Input: dimensioned drawing with shaded views. Units: mm. Origin: part minimum x, y, z. Give positions to 0.01 mm unless a question says otherwise; leave off trailing zeros. Loops run counter-clockwise (first coordinate to the right, second up) from the corner with the lowest first, then second, coordinate; pieces in that order, holes last.
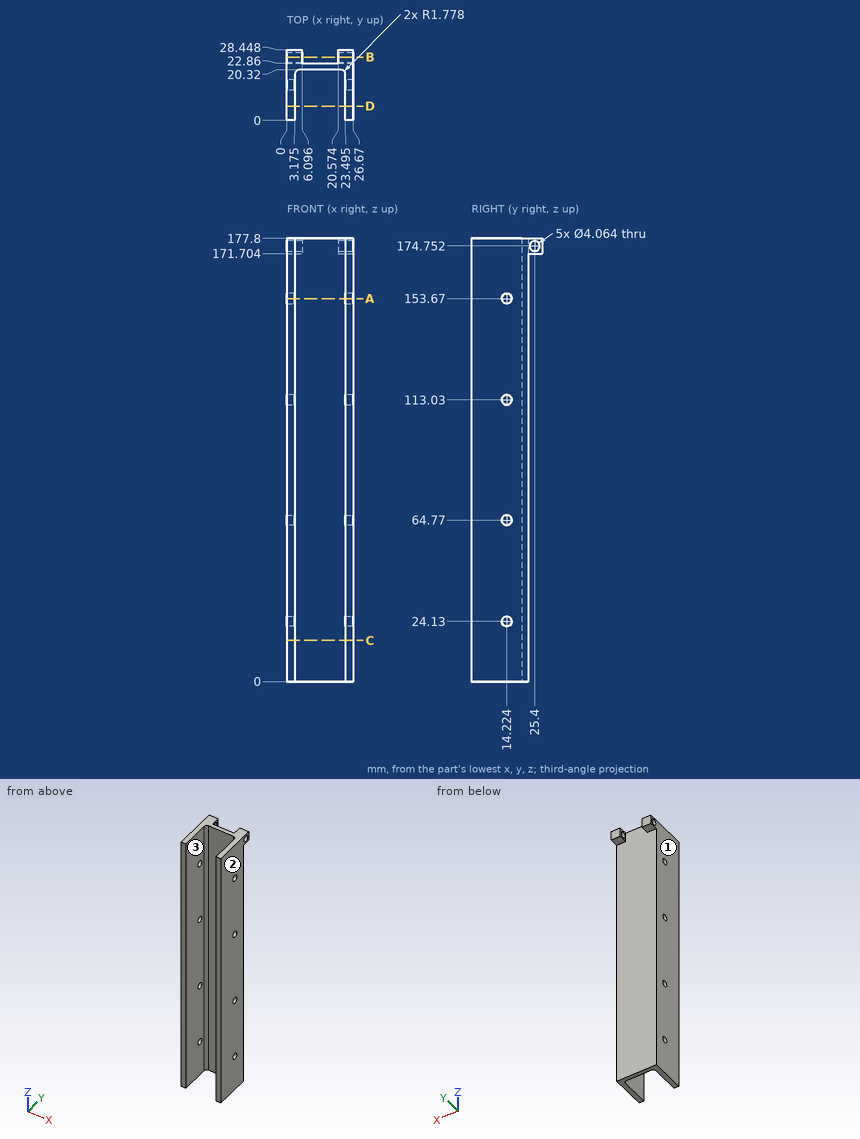
(1) First-contact query: pin 1 (8 mm diameter, centred on x = 19, z = 104.5, fed in from +Y); pin 2 (5 mm diameter, centred on x = 14, z = 116.5, fed in from -Y); pin 3 (1.7 mm diameter, centred on x = 2.5, y = 25.5, fed in from -Z). Flat tips, straight axial feed; report the tip coordinate or a pass-through.
A:
pin 1: stops at y = 22.86
pin 2: stops at y = 20.32
pin 3: stops at z = 171.7
(2) Section A-A, the plane z = 153.67. Return the cut outline in (x, y) (3 decimals), then the cut area to 3 significant figures.
A:
outline: (0, 0) - (3.175, 0) - (3.175, 12.192) - (0, 12.192) - close; (0, 16.256) - (3.175, 16.256) - (3.175, 18.542) arc R1.778 cw to (4.953, 20.32) - (21.717, 20.32) arc R1.778 cw to (23.495, 18.542) - (23.495, 16.256) - (26.67, 16.256) - (26.67, 22.86) - (0, 22.86) - close; (23.495, 0) - (26.67, 0) - (26.67, 12.192) - (23.495, 12.192) - close
area: 172 mm2
(3) Mould query, pull axis X, two halves, no side actions, for the marked faces 1, 2 and 3. Classes: pulls with the +X half, pulls with the -X half, needs draft (parallel to the pull), parting line crosses it, or undercut.
A:
face 1: pulls with the -X half
face 2: pulls with the +X half
face 3: undercut
(4) Section D-D, the plane y = 5.75. Return the cut outline in (x, z) (3 decimals), then the cut area to 3 significant figures.
A:
outline: (0, 0) - (3.175, 0) - (3.175, 177.8) - (0, 177.8) - close; (23.495, 0) - (26.67, 0) - (26.67, 177.8) - (23.495, 177.8) - close
area: 1,130 mm2
(5) Section C-C, the plane z = 16.5. Return the cut outline in (x, y) (3 decimals).
A:
outline: (0, 0) - (3.175, 0) - (3.175, 18.542) arc R1.778 cw to (4.953, 20.32) - (21.717, 20.32) arc R1.778 cw to (23.495, 18.542) - (23.495, 0) - (26.67, 0) - (26.67, 22.86) - (0, 22.86) - close
(6) Ray query, line 1 along Y through (x, z) = (1.3, 24.13); line 2 along X through (y, z) = (7.5, 107) (3 decimals); line 3 along Y through (x, z) = (10.5, 96). Return the intervals inside material, ascending.
A:
line 1: y = 0 to 12.19, 16.26 to 22.86
line 2: x = 0 to 3.175, 23.495 to 26.67
line 3: y = 20.32 to 22.86
(7) Section B-B, the plane y = 25.4. Return the cut outline in (x, z), then the cut area to 3 significant figures.
A:
outline: (0, 171.7) - (6.1, 171.7) - (6.1, 172.72) - (0, 172.72) - close; (0, 176.78) - (6.1, 176.78) - (6.1, 177.8) - (0, 177.8) - close; (20.57, 171.7) - (26.67, 171.7) - (26.67, 172.72) - (20.57, 172.72) - close; (20.57, 176.78) - (26.67, 176.78) - (26.67, 177.8) - (20.57, 177.8) - close
area: 24.8 mm2
